Check sheet for the modelled part. Datum: model origin and axes. Units: mm. A direction names the side the tool comes from. Give positions to 0.01 mm unless a question says otherwise; leave off trailing zeros. Order: outer loops, then holes, each group sorted by start corner. A loop starts at its lowest first (then second) coordinate and runs counter-clockwise, first axis right, second up. Notation, with made-up numbers: (14.25, 73.25) -> (52.25, 73.25) arc R21 ccw to (52.25, 106.25) -> close; hole circle Ø4 at (82, -10.75). An arc over 180 degrees is marked (long way). Write each question's results on one line, items separated by ' | '.
from build123d import *

# Parameters (mm, degrees)
SKETCH1_R           = 20.32
SKETCH1_R_2         = 12.7
BOSS_EXTRUDE1_DEPTH = 12.7
SKETCH2_W           = 3.175
SKETCH2_H           = 56.129579601
BOSS_EXTRUDE2_DEPTH = 38.1
CIRPATTERN1_COUNT   = 8


with BuildPart() as part:
    # Sketch1 → Boss-Extrude1 (new body)
    with BuildSketch(Plane(origin=(0, 0, 0), x_dir=(1, 0, 0), z_dir=(0, 1, 0))):
        Circle(SKETCH1_R)
        Circle(SKETCH1_R_2, mode=Mode.SUBTRACT)
    extrude(amount=BOSS_EXTRUDE1_DEPTH)

    # Sketch2 → Revolve1 (revolve)
    with BuildSketch(Plane(origin=(0, 6.35, 0), x_dir=(1, 0, 0), z_dir=(0, 1, 0))):
        with Locations((1.5875, 48.1352102)):
            Rectangle(SKETCH2_W, SKETCH2_H)
    revolve1 = revolve(axis=Axis((0, 6.35, -20.070420399), (0, 0, -1)))

    # Sketch4 → Boss-Extrude2 (add)
    with BuildSketch(Plane(origin=(0, 0, -63.5), x_dir=(-1, 0, 0), z_dir=(0, 0, -1))):
        with BuildLine():
            Line((-12.221045486, 0.123066306), (13.126308114, 13.038188042))
            Line((13.126308114, 13.038188042), (-6.337477412, 9.661472478))
            ThreePointArc((-6.337477412, 9.661472478), (-7.732958134, 9.047961526), (-8.681650548, 7.854753733))
            Line((-8.681650548, 7.854753733), (-12.221045486, 0.123066306))
        make_face()
    boss_extrude2 = extrude(amount=BOSS_EXTRUDE2_DEPTH)

    # CirPattern1: Revolve1, Boss-Extrude2 ×8 about axis
    cirpattern1_axis = Axis((0, 0, 0), (0, 1, 0))
    for i in range(1, CIRPATTERN1_COUNT):
        add(revolve1.rotate(cirpattern1_axis, i * 360 / CIRPATTERN1_COUNT))
        add(boss_extrude2.rotate(cirpattern1_axis, i * 360 / CIRPATTERN1_COUNT))


solid = part.part
1. Gauge pin test, flat ends, axial feed: pin 1 Ø1.4 at (x, y) = (-1.5, 5) entering from +Z; pin 2 Ø12 at (x, z) = (43.5, -4.5) entering from +Y (3 decimals); pin 3 Ø1.5 at (y, z) = (2, 69.5) entering from -X; pin 4 Ø2 at (x, y) = (44, 9.5) entering from +Z. Record the tip position at first contact, or that the pin passes through.
Verdict:
pin 1: stops at z = 101.6 | pin 2: stops at y = 9.525 | pin 3: stops at x = -11.71 | pin 4: stops at z = 56.08
2. Mould release check, pull along Z, two halves, no side actions. Record for faces 1 (the flat face through (-101.6, 8, -2)), 2 (the flat face through (60.68, 11.373, 55.687)), 3 (the flat face through (2, 8, -101.6)), 4 (the flat face through (-65.56, 4.04, 50.81)): +Z half, -Z half, draft (parallel to the pull), parting line (faces both ways), or undercut.
Verdict:
face 1: draft | face 2: +Z half | face 3: -Z half | face 4: undercut
3. Access from +Z, -Z, +X, -X, +Y, -Y to the whole of each face (thin tool, end or side, straight path). Record for faces 5 (the cylindrical face through (63.64, 9.06, -52.73)), 6 (the cylindrical face through (48.528, 4.204, -2.34)), 7 (the flat face through (-82.283, 11.373, 3.531)), 8 (the flat face through (10.43, 4.04, -82.28)).
Verdict:
face 5: +X, +Y | face 6: none | face 7: -X, +Y | face 8: -Z, +Y
4. Section check A-A on z = 0. Record the cut outline in (x, y) (3 decimals), then the cut area to 3 significant figures.
Verdict:
outline: (-101.6, 6.35) -> (-76.2, 6.35) -> (-76.2, 3.175) -> (-20.32, 3.175) -> (-20.32, 0) -> (-12.7, 0) -> (-12.7, 12.7) -> (-20.32, 12.7) -> (-20.32, 9.525) -> (-63.5, 9.525) -> (-63.5, 10.761) -> (-101.6, 10.761) -> close; (12.7, 0) -> (20.32, 0) -> (20.32, 3.175) -> (76.2, 3.175) -> (76.2, 6.35) -> (101.6, 6.35) -> (101.6, 10.761) -> (63.5, 10.761) -> (63.5, 9.525) -> (20.32, 9.525) -> (20.32, 12.7) -> (12.7, 12.7) -> close | area: 1,160 mm^2
5. Section check C-C on x = 27. Give the number of separate pieces and of enclosed holes in the cut face, then the cut area to 3 significant figures.
Verdict:
separate pieces: 3 | enclosed holes: 0 | area: 121 mm^2
6. Section check B-B on x = 0. Record the cut outline in (y, z) (3 decimals).
Verdict:
outline: (0, -20.32) -> (3.175, -20.32) -> (3.175, -76.2) -> (6.35, -76.2) -> (6.35, -101.6) -> (10.761, -101.6) -> (10.761, -63.5) -> (9.525, -63.5) -> (9.525, -20.32) -> (12.7, -20.32) -> (12.7, -12.7) -> (0, -12.7) -> close; (0, 12.7) -> (12.7, 12.7) -> (12.7, 20.32) -> (9.525, 20.32) -> (9.525, 63.5) -> (10.761, 63.5) -> (10.761, 101.6) -> (6.35, 101.6) -> (6.35, 76.2) -> (3.175, 76.2) -> (3.175, 20.32) -> (0, 20.32) -> close
7. Material ranges on probe 1 along Z at (x, y) = (0, 10); probe 2 along X at (y, z) = (9, 0); probe 3 along Z at (x, y) = (31, 5), recorded low to high. Write a range as from..to.
Verdict:
probe 1: z = -101.6..-63.5, -20.32..-12.7, 12.7..20.32, 63.5..101.6 | probe 2: x = -101.6..-12.7, 12.7..101.6 | probe 3: z = -35.06..-26.94, -2.87..2.87, 26.94..35.06
